Input: part model. Units: mm. Frame: model coordinates. A direction names the side the tool comes from. Give positions to 0.01 mm unless a question says otherwise; leave off trailing zeros. Order: outer loops, then holes, each group sorted by start corner. A loop starts at its lowest first (then second) coordinate and runs counter-clockwise, first axis right, second up. Notation, with made-up numbers: M -10.5,-34.75 L 5.5,-34.75 A16 cw 5.5,-12.75 Z; hole C 32.5,-31.75 d9. An arc over 180 degrees is marked long. Use a Markdown table: item, result.
from build123d import *

# Parameters (mm, degrees)
F0_W     = 9
F0_H     = 13
F1_DEPTH = 1.8
F2_DEPTH = 1
F3_DEPTH = 1
F4_DEPTH = 1
F5_DEPTH = 1
F7_DEPTH = 0.8
F8_W     = 3.2
F8_H     = 0.8
F9_DEPTH = 1
F10_R    = 0.39999
F11_SIZE = 0.4


# Not quite as in the source:
# - a fillet or chamfer is up to 0.001 mm smaller than in the source, because OpenCascade refuses the exact size
# - a feature names something its author has since deleted; it is built from what else it names


with BuildPart() as f1:
    # F0 (on Front) → F1 (new body)
    with BuildSketch(Plane.XZ):
        Polygon((-22, -22.5), (21.5, -22.5), (21.5, 22.5), (-22, 22.5), (-22, -7.5), align=None)
        with Locations((-16, -14.6)):
            Rectangle(F0_W, F0_H, mode=Mode.SUBTRACT)
        with Locations((-5.5, -14.6)):
            Rectangle(F0_W, F0_H, mode=Mode.SUBTRACT)
        with Locations((-16, -0.1)):
            Rectangle(F0_W, F0_H, mode=Mode.SUBTRACT)
        with Locations((-5.5, -0.1)):
            Rectangle(F0_W, F0_H, mode=Mode.SUBTRACT)
        with Locations((5, -14.6)):
            Rectangle(F0_W, F0_H, mode=Mode.SUBTRACT)
        with Locations((15.5, -14.6)):
            Rectangle(F0_W, F0_H, mode=Mode.SUBTRACT)
        with Locations((5, -0.1)):
            Rectangle(F0_W, F0_H, mode=Mode.SUBTRACT)
        with Locations((15.5, -0.1)):
            Rectangle(F0_W, F0_H, mode=Mode.SUBTRACT)
        with Locations((-16, 14.4)):
            Rectangle(F0_W, F0_H, mode=Mode.SUBTRACT)
        with Locations((-5.5, 14.4)):
            Rectangle(F0_W, F0_H, mode=Mode.SUBTRACT)
        with Locations((5, 14.4)):
            Rectangle(F0_W, F0_H, mode=Mode.SUBTRACT)
        with Locations((15.5, 14.4)):
            Rectangle(F0_W, F0_H, mode=Mode.SUBTRACT)
    extrude(amount=F1_DEPTH)

    # F2 (add): a face of the model
    f2_faces = [f1.faces().sort_by_distance(p)[0] for p in [
        (9.5, -0.9, -0.1),
    ]]
    extrude(f2_faces, amount=F2_DEPTH)

    # F3 (add): a face of the model
    f3_faces = [f1.faces().sort_by_distance(p)[0] for p in [
        (-10, -0.9, -0.1),
    ]]
    extrude(f3_faces, amount=F3_DEPTH)

    # F4 (add): faces of the model
    f4_faces = [f1.faces().sort_by_distance(p)[0] for p in [
        (-5, -0.9, 6.4),
        (4.5, -0.9, 6.4),
    ]]
    extrude(f4_faces, amount=F4_DEPTH)

    # F5 (add): faces of the model
    f5_faces = [f1.faces().sort_by_distance(p)[0] for p in [
        (-5, -0.9, -6.6),
        (4.5, -0.9, -6.6),
    ]]
    extrude(f5_faces, amount=F5_DEPTH)

    # F6 (on face) → F7 (cut)
    with BuildSketch(Plane.XZ.offset(1.8)):
        Polygon((5.2, -7.5), (5.2, -6.7), (-5.8, -6.7), (-5.8, -7.5), (-0.25, -7.5), align=None)
        Polygon((-9, -6.7), (-10.05, -6.7), (-10.45, -6.7), (-10.45, -7.5), (-9, -7.5), align=None)
        Polygon((9.5, 6.1155543663), (9.5, -6.7), (8.4, -6.7), (8.4, -7.5), (9.95, -7.5), (9.95, 6.5155543663), (-10.45, 6.5155543663), (-10.45, -6.7), (-10.05, -6.7), (-10.05, 6.1155543663), align=None)
    extrude(amount=-F7_DEPTH, mode=Mode.SUBTRACT)

    # F8 (on face) → F9 (join)
    with BuildSketch(Plane.XZ.offset(1.8)):
        with Locations((6.8, -7.1)):
            Rectangle(F8_W, F8_H)
        with Locations((-7.4, -7.1)):
            Rectangle(F8_W, F8_H)
    extrude(amount=F9_DEPTH)

    # F10 (radius 0.4 in the source; OpenCascade refuses exactly that, so slightly less here)
    f10_edges = [f1.edges().sort_by_distance(p)[0] for p in [
        (6.8, -2.8, -6.7),
        (6.8, -2.8, -7.5),
        (-7.4, -2.8, -7.5),
        (-7.4, -2.8, -6.7),
    ]]
    fillet(f10_edges, radius=F10_R)

    # F11
    f11_edges = [f1.edges().sort_by_distance(p)[0] for p in [
        (-20.5, -1.8, 14.4),
        (-11.5, -1.8, 14.4),
        (-16, -1.8, 20.9),
        (-16, -1.8, 7.9),
        (-16, -1.8, 6.4),
        (-20.5, -1.8, -0.1),
        (-16, -1.8, -6.6),
        (-11.5, -1.8, -0.1),
        (-5.5, -1.8, 7.9),
        (-10, -1.8, 14.4),
        (-1, -1.8, 14.4),
        (0.5, -1.8, 14.4),
        (5, -1.8, 7.9),
        (9.5, -1.8, 14.4),
        (-5, -1.8, 5.4),
        (-9, -1.8, -0.1),
        (-1, -1.8, -0.1),
        (0.5, -1.8, -0.1),
        (4.5, -1.8, 5.4),
        (8.5, -1.8, -0.1),
        (4.5, -1.8, -5.6),
        (-5, -1.8, -5.6),
        (-5.5, -1.8, 20.9),
        (5, -1.8, 20.9),
        (15.5, -1.8, 20.9),
        (20, -1.8, 14.4),
        (15.5, -1.8, 7.9),
        (11, -1.8, 14.4),
        (15.5, -1.8, 6.4),
        (11, -1.8, -0.1),
        (20, -1.8, -0.1),
        (15.5, -1.8, -6.6),
        (15.5, -1.8, -8.1),
        (11, -1.8, -14.6),
        (15.5, -1.8, -21.1),
        (20, -1.8, -14.6),
        (9.5, -1.8, -14.6),
        (5, -1.8, -8.1),
        (0.5, -1.8, -14.6),
        (5, -1.8, -21.1),
        (-5.5, -1.8, -21.1),
        (-1, -1.8, -14.6),
        (-5.5, -1.8, -8.1),
        (-10, -1.8, -14.6),
        (-11.5, -1.8, -14.6),
        (-16, -1.8, -8.1),
        (-20.5, -1.8, -14.6),
        (-16, -1.8, -21.1),
    ]]
    chamfer(f11_edges, length=F11_SIZE)


solid = f1.part
1) Cut plane B-B on x = 12. Return loops of the section in (y, z), and give its area (3 significant figures).
Response values:
| item | result |
|---|---|
| outline | M -1.8,-22.5 L 0,-22.5 L 0,-21.1 L -1.4,-21.1 L -1.8,-21.5 Z; M -1.8,-7.7 L -1.4,-8.1 L 0,-8.1 L 0,-6.6 L -1.4,-6.6 L -1.8,-7 Z; M -1.8,6.8 L -1.4,6.4 L 0,6.4 L 0,7.9 L -1.4,7.9 L -1.8,7.5 Z; M -1.8,21.3 L -1.4,20.9 L 0,20.9 L 0,22.5 L -1.8,22.5 Z |
| area | 10.3 mm² |
2) Reachability of faces 1 (the face through (-0.3, -1.8, -1.3)), 2 (the face through (-1, -1, -15)) from +Z, -Z, +X, -X, +Y, -Y: full face, straight path, thin tool, end or side. Return the list, or none.
Response values:
| item | result |
|---|---|
| face 1 | +Z, +X, -X, -Y |
| face 2 | +Y, -Y |
3) Cut plane A-A on z = 15. Return loops of the section in (x, y).
Response values:
| item | result |
|---|---|
| outline | M -22,-1.8 L -20.9,-1.8 L -20.5,-1.4 L -20.5,0 L -22,0 Z; M -11.5,-1.4 L -11.1,-1.8 L -10.4,-1.8 L -10,-1.4 L -10,0 L -11.5,0 Z; M -1,-1.4 L -0.6,-1.8 L 0.1,-1.8 L 0.5,-1.4 L 0.5,0 L -1,0 Z; M 9.5,-1.4 L 9.9,-1.8 L 10.6,-1.8 L 11,-1.4 L 11,0 L 9.5,0 Z; M 20,-1.4 L 20.4,-1.8 L 21.5,-1.8 L 21.5,0 L 20,0 Z |
4) Material intervals for line 1 (X direction, y = -0.3, z = 16.5); line 2 (Z direction, x = 8, y = -0.95); line 3 (Z direction, x = 15.5, y = -0.75), sorted ascending. Write a range as from..to.
Response values:
| item | result |
|---|---|
| line 1 | x = -22..-20.5, -11.5..-10, -1..0.5, 9.5..11, 20..21.5 |
| line 2 | z = -22.5..-21.1, -8.1..-5.6, 5.4..7.9, 20.9..22.5 |
| line 3 | z = -22.5..-21.1, -8.1..-6.6, 6.4..7.9, 20.9..22.5 |
5) Cut plane C-C on x = -2. State how many separate pieces and enclosed holes the cut face has, and give its area (3 significant figures).
Response values:
| item | result |
|---|---|
| separate pieces | 4 |
| enclosed holes | 0 |
| area | 13.0 mm² |
6) Mould query, pull axis Z, two halves, no side actions, for faces 3 (the face through (0, -1, 22.5)), 4 (the face through (-22, -1, 0)), 5 (the face through (0.5, -1, 14)), 6 (the face through (15, -1, 7.9)). Classes: released by +Z, released by -Z, zero draft, split by the parting line, or undercut.
Response values:
| item | result |
|---|---|
| face 3 | released by +Z |
| face 4 | zero draft |
| face 5 | undercut |
| face 6 | undercut |
7) First-contact query: pin 1 Ø8 at (x, z) = (-11.5, -17.5) entering from -Y. Flat tip, straight axial feed; report the tip coordinate or a pass-through.
Response values:
| item | result |
|---|---|
| pin 1 | stops at y = -1.8 |
